Geometry check sheet. Reference: the model listing, model coordinates, mm. Give positions to 0.01 mm unless a question says otherwise; leave off trailing zeros. Write each loop counter-clockwise with the first axis right and the second up, starting at its lowest first coordinate (ties: lowest second). Pieces come first, ordered by that corner, then holes. Notation, with made-up numbers: (62, 77) - (93, 77) arc R8 ccw to (93, 84) - close; hole circle Ø1 at (47, 46). An arc over 180 degrees is marked (long way). Write item = value, one per line. Start each with the question number.
(1) Depth check by flat-ended pin: pin 1 Ø1 at (y, z) = (11, -3) entering from +X; pin 2 Ø1.5 at (y, z) = (11, -10.5) entering from -X; pin 3 Ø6 at (y, z) = (17.5, -8) entering from +X. Enter the tip coordinate at first touch or a pass-through.
(2) Section check B-B, the plane z = -5. Enter the section's corners in (x, y), plus the area to 3 significant figures.
(3) Section check C-C, the plane y = 11.5. Enter the section's corners in (x, z), plus the area to 3 significant figures.
(4) Section check A-A, the plane x = -25. Enter the section's corners in (y, z).
(5) Thickness scan on L1, parallel to X at y = 3.5, z = -8; L2, parallel to X at y = 9.5, z = -8.75; L3, parallel to Y at x = -25, z = -8. Record the ranges inside material, lowest first.
(6) Section check D-D, the plane y = 17.5. Enter the section's corners in (x, z).
(7) Draft check along Y on faces 1 (the flat face through (-14.5, 8.1, 0)), 2 (the cylindrical face through (-15.24, 9.77, -5.92)), 3 (the flat face through (-32.2, 14.5, -5.9)), 4 (the flat face through (-9.723, 1.431, -5.916)). Enter one of: pulls with the +Y half, pulls with the -Y half, needs draft (parallel to the pull), parting line crosses it, or undercut.
```python
from build123d import *

# Parameters (mm, degrees)
SKETCH1_R           = 6
BOSS_EXTRUDE1_DEPTH = 12


with BuildPart() as part:
    # Sketch1 → Boss-Extrude1 (new body)
    with BuildSketch(Plane.XY):
        Polygon((-13.390210882, -4.996930009), (-5.952575928, 8.042282782), (-13.526047972, 21.003069991), (-28.537154971, 20.924644411), (-35.974789926, 7.885431621), (-28.401317881, -5.075355589), align=None)
        with Locations((-20.963682927, 7.963857201)):
            Circle(SKETCH1_R, mode=Mode.SUBTRACT)
    extrude(amount=-BOSS_EXTRUDE1_DEPTH)


solid = part.part
```
Model answer:
q1.pin_1 = -7.39
q1.pin_2 = -34.63
q1.pin_3 = -9.73
q2.outline = (-35.97, 7.89) - (-28.4, -5.08) - (-13.39, -5) - (-5.95, 8.04) - (-13.53, 21) - (-28.54, 20.92) - close; hole circle Ø12 at (-20.96, 7.96)
q2.area = 472 mm²
q3.outline = (-33.91, -12) - (-25.81, -12) - (-25.81, 0) - (-33.91, 0) - close; (-16.12, -12) - (-7.97, -12) - (-7.97, 0) - (-16.12, 0) - close
q3.area = 195 mm²
q4.outline = (-5.06, -12) - (3.52, -12) - (3.52, 0) - (-5.06, 0) - close; (12.4, -12) - (20.94, -12) - (20.94, 0) - (12.4, 0) - close
q5.L1 = -33.41 to -24.97, -16.95 to -8.54
q5.L2 = -35.05 to -26.76, -15.16 to -6.8
q5.L3 = -5.06 to 3.52, 12.4 to 20.94
q6.outline = (-30.49, -12) - (-11.48, -12) - (-11.48, 0) - (-30.49, 0) - close
q7.face_1 = needs draft
q7.face_2 = undercut
q7.face_3 = pulls with the +Y half
q7.face_4 = pulls with the -Y half
